from build123d import *

# Parameters (mm, degrees)
F1_DEPTH = 3.175
F2_D     = 4.7625
F3_D     = 4.7625


with BuildPart() as f1:
    # F0 (on Front) → F1 (new body)
    with BuildSketch(Plane.XZ):
        with BuildLine():
            Line((40.6890114234, 6.6018716117), (-37.1726150847, 6.6018716117))
            ThreePointArc((-37.1726150847, 6.6018716117), (-36.5382474018, 5.0703725481), (-36.3218763988, 3.4268716117))
            ThreePointArc((-36.3218763988, 3.4268716117), (-36.5382474018, 1.7833706753), (-37.1726150847, 0.2518716117))
            Line((-37.1726150847, 0.2518716117), (40.6890110201, 0.2518716117))
            ThreePointArc((40.6890110201, 0.2518716117), (39.8382725358, 3.4268716658), (40.6890114234, 6.6018716117))
        make_face()
        with BuildLine():
            Line((-37.1726150847, 6.6018716117), (-42.6718763988, 6.6018716117))
            Line((-42.6718763988, 6.6018716117), (-42.6718763988, 0.2518716117))
            Line((-42.6718763988, 0.2518716117), (-37.1726150847, 0.2518716117))
            ThreePointArc((-37.1726150847, 0.2518716117), (-36.5382474018, 1.7833706753), (-36.3218763988, 3.4268716117))
            ThreePointArc((-36.3218763988, 3.4268716117), (-36.5382474018, 5.0703725481), (-37.1726150847, 6.6018716117))
        make_face()
        with BuildLine():
            Line((-42.6718763988, 0.2518716117), (-42.6718763988, 6.6018716117))
            Line((-42.6718763988, 6.6018716117), (-37.1726150847, 6.6018716117))
            ThreePointArc((-37.1726150847, 6.6018716117), (-49.0218763988, 3.4268716117), (-37.1726150847, 0.2518716117))
            Line((-37.1726150847, 0.2518716117), (-42.6718763988, 0.2518716117))
        make_face()
        with BuildLine():
            ThreePointArc((52.5382725358, 3.4268712625), (47.831773667, 9.5605002072), (40.6890114234, 6.6018716117))
            Line((40.6890114234, 6.6018716117), (46.2281236012, 6.6018716117))
            Line((46.2281236012, 6.6018716117), (46.2281236012, 0.2518716117))
            Line((46.2281236012, 0.2518716117), (40.6890110201, 0.2518716117))
            ThreePointArc((40.6890110201, 0.2518716117), (47.8317732774, -2.7067577866), (52.5382725358, 3.4268712625))
        make_face()
        with BuildLine():
            Line((46.2281236012, 6.6018716117), (40.6890114234, 6.6018716117))
            ThreePointArc((40.6890114234, 6.6018716117), (39.8382725358, 3.4268716658), (40.6890110201, 0.2518716117))
            Line((40.6890110201, 0.2518716117), (46.2281236012, 0.2518716117))
            Line((46.2281236012, 0.2518716117), (46.2281236012, 6.6018716117))
        make_face()
    extrude(amount=F1_DEPTH)

    # F2 (through all)
    with Locations(Plane(origin=(0, 0, 0), x_dir=(1, 0, 0), z_dir=(0, 1, 0))):
        with Locations((-42.6718763988, -3.4268716117)):
            Hole(F2_D / 2)

    # F3 (through all)
    with Locations(Plane(origin=(0, 0, 0), x_dir=(1, 0, 0), z_dir=(0, 1, 0))):
        with Locations((46.1882725358, -3.4268712625)):
            Hole(F3_D / 2)


solid = f1.part
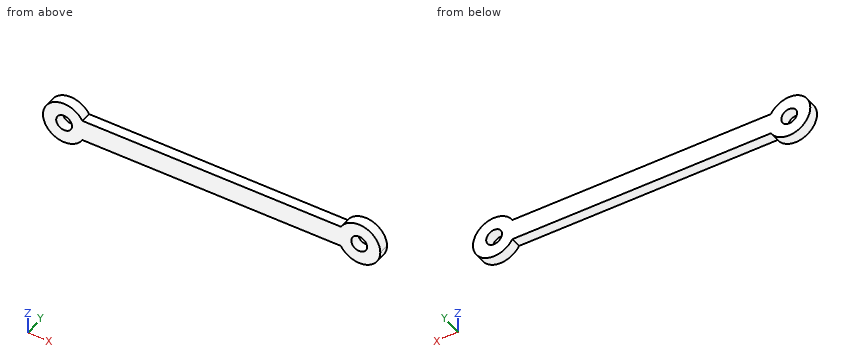
Geometry: final body of the model. Coordinates: model frame, mm. Round coordinates to 2 decimals unless told otherwise and drop trailing zeros. Order: outer loops, then holes, each group sorted by start corner. A loop starts at its lowest first (then second) coordinate and runs counter-clockwise, first axis right, second up.
Q1. Section A-A, the plane y = -0.85. Output: boundary loops of the cut face in (x, z).
Result sheet:
outline: (-37.17, 0.25) - (40.69, 0.25) arc R6.35 ccw (long way) to (40.69, 6.6) - (-37.17, 6.6) arc R6.35 ccw (long way) to start; hole circle Ø4.76 at (-42.67, 3.43); hole circle Ø4.76 at (46.19, 3.43)
Q2. Section B-B, the plane z = -0.75. Output: boundary loops of the cut face in (x, y) (3 decimals).
Result sheet:
outline: (-47.455, -3.175) - (-37.889, -3.175) - (-37.889, 0) - (-47.455, 0) - close; (41.405, -3.175) - (50.971, -3.175) - (50.971, 0) - (41.405, 0) - close
Q3. Pin query (flat end, axial travel): pin 1 (1.5 mm diameter, centred on x = 40.5, y = -1, fed in from -Z); pin 2 (5.5 mm diameter, centred on x = 46.19, z = 3.43, fed in from -Y) (3 decimals); pin 3 (1.5 mm diameter, centred on x = -9.5, y = -2.5, fed in from +Z); pin 4 (1.5 mm diameter, centred on y = -1, z = 4.5, fed in from +X). Return the tip coordinate at first contact, or that it passes through.
Result sheet:
pin 1: stops at z = -0.57
pin 2: stops at y = -3.175
pin 3: stops at z = 6.6
pin 4: stops at x = 52.53
Q4. Material intervals for probe 1 along X at (y, z) = (-2, 1.25); probe 2 along X at (y, z) = (-0.65, 2); probe 3 along Z at (x, y) = (-19, -1.7), sorted ascending.
Result sheet:
probe 1: x = -48.64 to -43.64, -41.71 to 45.22, 47.15 to 52.15
probe 2: x = -48.86 to -44.58, -40.77 to 44.28, 48.09 to 52.38
probe 3: z = 0.25 to 6.6
Q5. Section C-C, the plane x = -9. Output: boundary loops of the cut face in (y, z) (3 decimals).
Result sheet:
outline: (-3.175, 0.252) - (0, 0.252) - (0, 6.602) - (-3.175, 6.602) - close
